from build123d import *

# Parameters (mm, degrees)
BOSS_EXTRUDE1_DEPTH = 134.9375
SKETCH4_W           = 25.4
SKETCH4_H           = 19.05
CUT_EXTRUDE1_DEPTH  = 6.35
SKETCH6_R           = 2.921
CUT_EXTRUDE3_DEPTH  = 25.4
BOSS_EXTRUDE2_DEPTH = 38.1
CUT_EXTRUDE4_DEPTH  = 143.860280702


with BuildPart() as part:
    # Sketch3 → Boss-Extrude1 (new body)
    with BuildSketch(Plane(origin=(0, 0, 0), x_dir=(0, 0, -1), z_dir=(1, 0, 0))):
        with BuildLine():
            Line((0, 0), (95.25, 0))
            Line((95.25, 0), (95.25, 44.45))
            ThreePointArc((95.25, 44.45), (49.555547135, 18.088113282), (0, 0))
        make_face()
    extrude(amount=BOSS_EXTRUDE1_DEPTH)

    # Sketch4 → Cut-Extrude1 (cut)
    with BuildSketch(Plane(origin=(134.9375, 0, 0), x_dir=(0, 0, -1), z_dir=(1, 0, 0))):
        with Locations((82.55, 17.145)):
            Rectangle(SKETCH4_W, SKETCH4_H)
    extrude(amount=-CUT_EXTRUDE1_DEPTH, mode=Mode.SUBTRACT)

    # Sketch6 → Cut-Extrude3 (cut)
    with BuildSketch(Plane(origin=(128.5875, 0, 0), x_dir=(0, 0, -1), z_dir=(1, 0, 0))):
        with Locations((82.55, 17.145)):
            Circle(SKETCH6_R)
    extrude(amount=-CUT_EXTRUDE3_DEPTH, mode=Mode.SUBTRACT)

    # Sketch7 → Boss-Extrude2 (add)
    with BuildSketch(Plane.XZ):
        Polygon((0, -82.55), (-7.922780702, -83.947), (-7.922780702, -71.12), (0, -72.517), align=None)
        Polygon((0, -62.780333333), (-7.922780702, -64.177333333), (-7.922780702, -51.350333333), (0, -52.747333333), align=None)
        Polygon((0, -43.010666667), (-7.922780702, -44.407666667), (-7.922780702, -31.580666667), (0, -32.977666667), align=None)
        Polygon((0, -23.241), (-7.922780702, -24.638), (-7.922780702, -11.811), (0, -13.208), align=None)
    extrude(amount=-BOSS_EXTRUDE2_DEPTH)

    # Sketch8 → Cut-Extrude4 (cut, through all)
    with BuildSketch(Plane(origin=(134.9375, 0, 0), x_dir=(0, 0, -1), z_dir=(1, 0, 0))):
        with BuildLine():
            Line((95.25, 44.45), (0, 44.45))
            Line((0, 44.45), (0, 0))
            ThreePointArc((0, 0), (49.555547135, 18.088113282), (95.25, 44.45))
        make_face()
    extrude(amount=-CUT_EXTRUDE4_DEPTH, mode=Mode.SUBTRACT)


solid = part.part
Input: part model. Units: mm. Frame: model coordinates. A direction names the side the tool comes from. Coordinates: 2 decimals unless noted, no trailing zeros. Loops run counter-clockwise (first coordinate to the right, second up) from the corner with the lowest first, then second, coordinate; pieces in that order, holes last.
(1) Set-up query: faces 1 (the face through (128.588, 19, -80)), 2 (the face through (-3.91, 3.83, -23.93)), 3 (the face through (-3.91, 18.2, -83.24)), 4 (the face through (103.188, 17, -83)). Return all of +Z, -Z, +X, -X, +Y, -Y with unobstructed straight access to the full face (end or side cutting, diameter ignored); none if empty.
(2) Section C-C on z = -7. Return the cut outline in (x, y), then the cut area to 3 significant figures.
(3) Section B-B on z = -37. Return the cut outline in (x, y), then the cut area to 3 significant figures.
(4) First-contact query: pin 1 Ø3 at (x, y) = (132, 20.5) entering from -Z; pin 2 Ø1.8 at (y, z) = (18.5, -81) entering from +X; pin 3 Ø3 at (x, z) = (132, -88.5) entering from +Y. Flat tips, straight axial feed; report the tip coordinate or a pass-through.
(5) Section A-A on x = 94.5. Return the cut outline in (y, z).
(6) Pull-direction query (Z, two-part tool) for faces 5 (the face through (-4.02, 5.39, -32.27)), 6 (the face through (132, 7.62, -82)), 7 (the face through (67, 22, -95.25)); classes: released by +Z, released by -Z, zero draft, split by the parting line, or undercut.
(7) Material intervals for probe 1 along X at (y, z) = (21, -86.5); probe 2 along Y at (x, z) = (118, -82.55); probe 3 along Y at (x, z) = (116, -82), sorted ascending.
Data:
1. face 1: -Z, +X
1. face 2: +Y, -Y
1. face 3: -Z, +Y, -Y
1. face 4: +X
2. outline: (0, 0) - (134.94, 0) - (134.94, 1.98) - (0, 1.98) - close
2. area: 267 mm2
3. outline: (-7.92, 0) - (134.94, 0) - (134.94, 12.57) - (-7.92, 12.57) - close
3. area: 1,800 mm2
4. pin 1: stops at z = -69.85
4. pin 2: stops at x = 128.59
4. pin 3: stops at y = 40.86
5. outline: (0, -95.25) - (44.45, -95.25) arc R304.8 cw to (0, 0) - close
6. face 5: undercut
6. face 6: zero draft
6. face 7: released by -Z
7. probe 1: x = 0 to 128.59
7. probe 2: y = 0 to 14.22, 20.07 to 36.04
7. probe 3: y = 0 to 14.28, 20.01 to 35.7
